Model file for the job. Use its own axes, mm. Face numbers are marked on the shaded views. A direction names the side the tool comes from. Coordinates: 2 decimals unless noted, no trailing zeros. Write each loop counter-clockwise with the first axis right and the second up, starting at its lowest first coordinate (ties: lowest second). Pieces come first, ordered by that corner, then holes. Notation, with made-up numbers: M 48.5,13.25 L 95.5,13.25 A14 ccw 95.5,23.25 Z; hole C 47,-18 d10. An arc over 180 degrees is marked long. One line per question, with ' | ' between items. Start each with the question number.
(1) Two-plate mould, pull along X, no slides. Class the marked faces 1, 2 and 3: +X half, -X half, draft (parallel to the pull), parting line (faces both ways), or undercut.
(2) Cut at D-D (z = 9.5). Write the cut outline in (x, y).
(3) Wall check: probe 1 along Y at (x, z) = (-22, 1.5); probe 2 along X at (y, z) = (-4.5, 8.75); probe 3 along X at (y, z) = (0, 1.6). Give the ranges that are in metal, low to high.
(4) Flat gauge pins, fed straight in: pin 1 Ø3 at (x, y) = (35, 25) entering from +Z; pin 2 Ø2.5 at (x, y) = (-22, 31) entering from +Z. Where does each tip first touch, or does it go through?
(5) Tool access for the marked faces 4 and 5: list every direction of +Z, -Z, +X, -X, +Y, -Y with a clear straight run to the whole face (end or side of a thin tool).
(6) Cut at A-A (z = 14.6). Write the cut outline in (x, y) (3 decimals), plus the area to 3 significant figures.
(7) Cut at B-B (y = -31). Write the cut outline in (x, z), plus the area to 3 significant figures.
(8) Cut at C-C (x = 54). Write the cut outline in (y, z).
from build123d import *

# Parameters (mm, degrees)
SKETCH1_W           = 114.5
SKETCH1_H           = 75.2
BOSS_EXTRUDE1_DEPTH = 3
CUT_EXTRUDE1_REACH  = 83.282
SKETCH3_R           = 1.35
SKETCH5_W           = 3
SKETCH5_H           = 75.2
BOSS_EXTRUDE3_DEPTH = 17.6
CUT_EXTRUDE2_REACH  = 124.264
CUT_EXTRUDE3_REACH  = 124.264
CUT_EXTRUDE4_REACH  = 121.459
CUT_EXTRUDE5_REACH  = 121.459
CUT_EXTRUDE6_REACH  = 124.264
SKETCH10_R          = 2.425
CUT_EXTRUDE7_REACH  = 124.264
SKETCH11_R          = 1.4
CHAMFER1_SIZE       = 2


with BuildPart() as part:
    # Sketch1 → Boss-Extrude1 (new body)
    with BuildSketch(Plane.XY):
        with Locations((14.75, 0)):
            Rectangle(SKETCH1_W, SKETCH1_H)
    extrude(amount=BOSS_EXTRUDE1_DEPTH)

    # Sketch3 → Cut-Extrude1 (cut, up to next)
    with BuildSketch(Plane.XY, mode=Mode.PRIVATE) as cut_extrude1_sk1:
        with Locations(Location((35, 25, 0), (0, 0, 180))):
            Circle(SKETCH3_R)
    cut_extrude1_tool1 = extrude(cut_extrude1_sk1.sketch, amount=CUT_EXTRUDE1_REACH, mode=Mode.PRIVATE) & part.part
    # Sketch3 → Cut-Extrude1 (cut, up to next)
    with BuildSketch(Plane.XY, mode=Mode.PRIVATE) as cut_extrude1_sk2:
        with Locations(Location((-22, 31, 0), (0, 0, 180))):
            Circle(SKETCH3_R)
    cut_extrude1_tool2 = extrude(cut_extrude1_sk2.sketch, amount=CUT_EXTRUDE1_REACH, mode=Mode.PRIVATE) & part.part
    # Sketch3 → Cut-Extrude1 (cut, up to next)
    with BuildSketch(Plane.XY, mode=Mode.PRIVATE) as cut_extrude1_sk3:
        with Locations(Location((-22, -31, 0), (0, 0, 180))):
            Circle(SKETCH3_R)
    cut_extrude1_tool3 = extrude(cut_extrude1_sk3.sketch, amount=CUT_EXTRUDE1_REACH, mode=Mode.PRIVATE) & part.part
    # Sketch3 → Cut-Extrude1 (cut, up to next)
    with BuildSketch(Plane.XY, mode=Mode.PRIVATE) as cut_extrude1_sk4:
        with Locations(Location((35, -25, 0), (0, 0, 180))):
            Circle(SKETCH3_R)
    cut_extrude1_tool4 = extrude(cut_extrude1_sk4.sketch, amount=CUT_EXTRUDE1_REACH, mode=Mode.PRIVATE) & part.part
    # Sketch3 → Cut-Extrude1 (cut, up to next)
    with BuildSketch(Plane.XY, mode=Mode.PRIVATE) as cut_extrude1_sk5:
        with BuildLine():
            Line((37.352968819, -11.360132143), (33.626035358, -17.571687912))
            Line((33.626035358, -17.571687912), (42.200964615, -22.716645466))
            Line((42.200964615, -22.716645466), (45.927898076, -16.505089698))
            ThreePointArc((45.927898076, -16.505089698), (58.746427842, 14.577379737), (37.352968819, -11.360132143))
        make_face()
    cut_extrude1_tool5 = extrude(cut_extrude1_sk5.sketch, amount=CUT_EXTRUDE1_REACH, mode=Mode.PRIVATE) & part.part
    # Sketch3 → Cut-Extrude1 (cut, up to next)
    with BuildSketch(Plane.XY, mode=Mode.PRIVATE) as cut_extrude1_sk6:
        Polygon((15, -37.6), (72, -14.6), (72, -37.6), align=None)
    cut_extrude1_tool6 = extrude(cut_extrude1_sk6.sketch, amount=CUT_EXTRUDE1_REACH, mode=Mode.PRIVATE) & part.part
    # Sketch3 → Cut-Extrude1 (cut, up to next)
    with BuildSketch(Plane.XY, mode=Mode.PRIVATE) as cut_extrude1_sk7:
        Polygon((15, 37.6), (72, 14.6), (72, 37.6), align=None)
    cut_extrude1_tool7 = extrude(cut_extrude1_sk7.sketch, amount=CUT_EXTRUDE1_REACH, mode=Mode.PRIVATE) & part.part
    add(cut_extrude1_tool1.solids().sort_by_distance((35, 25, 0))[0], mode=Mode.SUBTRACT)
    add(cut_extrude1_tool2.solids().sort_by_distance((-22, 31, 0))[0], mode=Mode.SUBTRACT)
    add(cut_extrude1_tool3.solids().sort_by_distance((-22, -31, 0))[0], mode=Mode.SUBTRACT)
    add(cut_extrude1_tool4.solids().sort_by_distance((35, -25, 0))[0], mode=Mode.SUBTRACT)
    add(cut_extrude1_tool5.solids().sort_by_distance((49.284681, -1.192198, 0))[0], mode=Mode.SUBTRACT)
    add(cut_extrude1_tool6.solids().sort_by_distance((53, -29.933333, 0))[0], mode=Mode.SUBTRACT)
    add(cut_extrude1_tool7.solids().sort_by_distance((53, 29.933333, 0))[0], mode=Mode.SUBTRACT)

    # Sketch5 → Boss-Extrude3 (add)
    with BuildSketch(Plane.XY.offset(3)):
        Polygon((72, -14.6), (69, -15.810526316), (69, 15.810526316), (72, 14.6), align=None)
        with Locations((-41, 0)):
            Rectangle(SKETCH5_W, SKETCH5_H)
    extrude(amount=BOSS_EXTRUDE3_DEPTH)

    # Sketch6 → Cut-Extrude2 (cut, up to next)
    with BuildSketch(Plane.ZY.offset(42.5), mode=Mode.PRIVATE) as cut_extrude2_sk1:
        with BuildLine():
            Line((3, 37.6), (19.996596859, 2.62235435))
            ThreePointArc((19.996596859, 2.62235435), (20.447203655, 1.345440234), (20.6, 0))
            Line((20.6, 0), (20.6, 37.6))
            Line((20.6, 37.6), (3, 37.6))
        make_face()
    cut_extrude2_tool1 = extrude(cut_extrude2_sk1.sketch, amount=-CUT_EXTRUDE2_REACH, mode=Mode.PRIVATE) & part.part
    add(cut_extrude2_tool1.solids().sort_by_distance((-42.5, 25.516122, 14.735887))[0], mode=Mode.SUBTRACT)

    # Sketch7 → Cut-Extrude3 (cut, up to next)
    with BuildSketch(Plane.ZY.offset(42.5), mode=Mode.PRIVATE) as cut_extrude3_sk1:
        with BuildLine():
            Line((20.6, 0), (20.6, -37.6))
            Line((20.6, -37.6), (3, -37.6))
            Line((3, -37.6), (19.996596859, -2.62235435))
            ThreePointArc((19.996596859, -2.62235435), (20.447203655, -1.345440234), (20.6, 0))
        make_face()
    cut_extrude3_tool1 = extrude(cut_extrude3_sk1.sketch, amount=-CUT_EXTRUDE3_REACH, mode=Mode.PRIVATE) & part.part
    add(cut_extrude3_tool1.solids().sort_by_distance((-42.5, -25.516122, 14.735887))[0], mode=Mode.SUBTRACT)

    # Sketch8 → Cut-Extrude4 (cut, up to next)
    with BuildSketch(Plane.ZY.offset(-69), mode=Mode.PRIVATE) as cut_extrude4_sk1:
        with BuildLine():
            Line((18.119604827, 4.859257336), (3, 15.810526316))
            Line((3, 15.810526316), (20.6, 15.810526316))
            Line((20.6, 15.810526316), (20.6, 0))
            ThreePointArc((20.6, 0), (19.944044768, 2.727853647), (18.119604827, 4.859257336))
        make_face()
    cut_extrude4_tool1 = extrude(cut_extrude4_sk1.sketch, amount=-CUT_EXTRUDE4_REACH, mode=Mode.PRIVATE) & part.part
    add(cut_extrude4_tool1.solids().sort_by_distance((69, 11.454378, 14.798599))[0], mode=Mode.SUBTRACT)

    # Sketch9 → Cut-Extrude5 (cut, up to next)
    with BuildSketch(Plane.ZY.offset(-69), mode=Mode.PRIVATE) as cut_extrude5_sk1:
        with BuildLine():
            Line((18.119604827, -4.859257336), (3, -15.810526316))
            Line((3, -15.810526316), (20.6, -15.810526316))
            Line((20.6, -15.810526316), (20.6, 0))
            ThreePointArc((20.6, 0), (19.944044768, -2.727853647), (18.119604827, -4.859257336))
        make_face()
    cut_extrude5_tool1 = extrude(cut_extrude5_sk1.sketch, amount=-CUT_EXTRUDE5_REACH, mode=Mode.PRIVATE) & part.part
    add(cut_extrude5_tool1.solids().sort_by_distance((69, -11.454378, 14.798599))[0], mode=Mode.SUBTRACT)

    # Sketch10 → Cut-Extrude6 (cut, up to next)
    with BuildSketch(Plane.ZY.offset(42.5), mode=Mode.PRIVATE) as cut_extrude6_sk1:
        with Locations(Location((14.6, 0, 0), (0, 0, 270))):
            Circle(SKETCH10_R)
    cut_extrude6_tool1 = extrude(cut_extrude6_sk1.sketch, amount=-CUT_EXTRUDE6_REACH, mode=Mode.PRIVATE) & part.part
    add(cut_extrude6_tool1.solids().sort_by_distance((-42.5, 0, 14.6))[0], mode=Mode.SUBTRACT)

    # Sketch11 → Cut-Extrude7 (cut, up to next)
    with BuildSketch(Plane(origin=(72, 0, 0), x_dir=(0, 0, -1), z_dir=(1, 0, 0)), mode=Mode.PRIVATE) as cut_extrude7_sk1:
        with Locations((-14.6, 0)):
            Circle(SKETCH11_R)
    cut_extrude7_tool1 = extrude(cut_extrude7_sk1.sketch, amount=-CUT_EXTRUDE7_REACH, mode=Mode.PRIVATE) & part.part
    add(cut_extrude7_tool1.solids().sort_by_distance((72, 0, 14.6))[0], mode=Mode.SUBTRACT)

    # Chamfer1
    # the kernel refuses this chamfer: 2 mm, written as the material it adds along each edge
    with BuildSketch(Plane(origin=(69, -20.953892292, 3), x_dir=(-0.9996219169112968, 0, -0.0274958766105862), z_dir=(0, 1, 0))) as chamfer1_piece_1_section:
        Polygon((CHAMFER1_SIZE * 0.999621916911, CHAMFER1_SIZE * 0.0274958766106), (-CHAMFER1_SIZE * 0.0274958766106, CHAMFER1_SIZE * 0.999621916911), (0, 0), align=None)
    chamfer1_piece_1 = extrude(amount=41.907784583, mode=Mode.PRIVATE)
    chamfer1_piece_1 = chamfer1_piece_1 - Plane(origin=(50, 0, 3.647655416), x_dir=(-0.23953540727459496, -0.9708876292660207, 0), z_dir=(0, 0, -1)) * Cylinder(17, 92, mode=Mode.PRIVATE)
    chamfer1_piece_1 = split(chamfer1_piece_1, bisect_by=Plane(origin=(68.334125846, -10.062431967, 10.935967533), z_dir=(0, 0.8098762227411254, -0.5866008044987383)), keep=Keep.TOP, mode=Mode.PRIVATE)
    chamfer1_piece_1 = split(chamfer1_piece_1, bisect_by=Plane(origin=(68.334125846, 10.062431967, 10.935967533), z_dir=(0, -0.8098762227411249, -0.5866008044987391)), keep=Keep.TOP, mode=Mode.PRIVATE)
    add(chamfer1_piece_1)
    with BuildSketch(Plane(origin=(-39.5, -37.6, 3), x_dir=(0.9996219169112968, 0, -0.027495876610586296), z_dir=(0, 1, 0))) as chamfer1_piece_2_section:
        Polygon((CHAMFER1_SIZE * 0.999621916911, -CHAMFER1_SIZE * 0.0274958766106), (-CHAMFER1_SIZE * 0.0274958766106, -CHAMFER1_SIZE * 0.999621916911), (0, 0), align=None)
    chamfer1_piece_2 = extrude(amount=75.2, mode=Mode.PRIVATE)
    chamfer1_piece_2 = split(chamfer1_piece_2, bisect_by=Plane(origin=(-38.832756729, 6.928738124, 17.904006933), z_dir=(0, -0.4370590583687447, -0.8994328098851111)), keep=Keep.TOP, mode=Mode.PRIVATE)
    chamfer1_piece_2 = split(chamfer1_piece_2, bisect_by=Plane(origin=(-38.832756729, -6.928738124, 17.904006933), z_dir=(0, 0.4370590583688008, -0.8994328098850838)), keep=Keep.TOP, mode=Mode.PRIVATE)
    add(chamfer1_piece_2)


solid = part.part
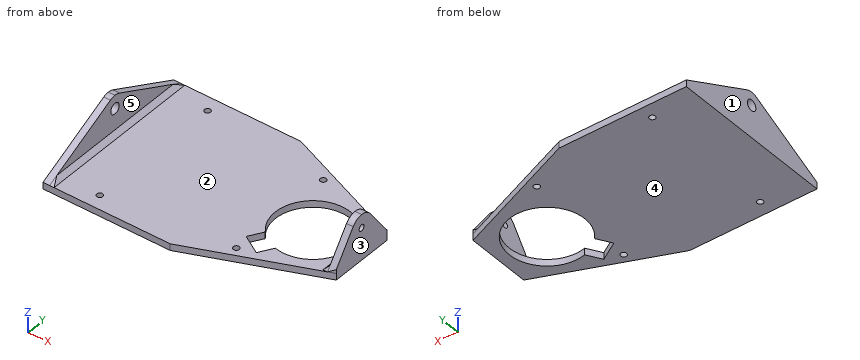
Filled in:
1) face 1: -X half | face 2: undercut | face 3: +X half
2) outline: M -42.5,-24.22 L -39.5,-24.22 L -39.5,24.22 L -42.5,24.22 Z; M 69,-11.1 L 72,-11.1 L 72,11.1 L 69,11.1 Z
3) probe 1: -37.6 to -32.35, -29.65 to 29.65, 32.35 to 37.6 | probe 2: -42.5 to -39.5, 69 to 72 | probe 3: -42.5 to 33, 67 to 72
4) pin 1: z = 3 | pin 2: through
5) face 4: -Z, +X, -X, +Y, -Y | face 5: +Z, +Y, -Y
6) outline: M -42.5,-13.728 L -39.5,-13.728 L -39.5,-2.425 L -42.5,-2.425 Z; M -42.5,2.425 L -39.5,2.425 L -39.5,13.728 L -42.5,13.728 Z; M 69,-7.409 L 72,-7.409 L 72,-1.4 L 69,-1.4 Z; M 69,1.4 L 72,1.4 L 72,7.409 L 69,7.409 Z | area: 104 mm²
7) outline: M -42.5,0 L -23.35,0 L -23.35,3 L -37.5,3 L -39.5,5 L -39.5,6.21 L -42.5,6.21 Z; M -20.65,0 L 31.36,0 L 31.36,3 L -20.65,3 Z | area: 225 mm²
8) outline: M -21.86,0 L -16.52,0 L -16.52,3 L -21.86,3 Z; M 16.52,0 L 21.86,0 L 21.86,3 L 16.52,3 Z
